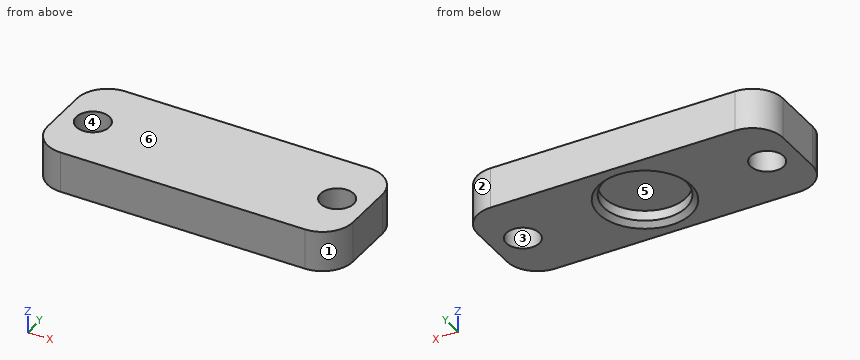
from build123d import *

# Parameters (mm, degrees)
SKETCH1_W                        = 95.25
SKETCH1_H                        = 34.925
BASE_FLANGE1_DEPTH               = 12.7
SKETCH2_R                        = 12.827
CUT_EXTRUDE1_DEPTH               = 4.7625
F_13_32_0_40625_DIAMETER_HOLE1_D = 10.31875
CHAMFER1_SIZE                    = 1.5875
FILLET1_R                        = 9.525


# Sheet-metal steps are written as plain solids
with BuildPart() as part:
    # Sketch1 → Base-Flange1 (new body)
    with BuildSketch(Plane.XY):
        Rectangle(SKETCH1_W, SKETCH1_H)
    extrude(amount=BASE_FLANGE1_DEPTH)

    # Sketch2 → Cut-Extrude1 (cut)
    with BuildSketch(Plane.XY):
        with Locations(Location((0, 0, 0), (0, 0, 180))):
            Circle(SKETCH2_R)
    extrude(amount=CUT_EXTRUDE1_DEPTH, mode=Mode.SUBTRACT)

    # 13/32 (0.40625) Diameter Hole1 (through all)
    with Locations(Plane.XY.offset(12.7)):
        with Locations((38.1, 0), (-38.1, 0)):
            Hole(F_13_32_0_40625_DIAMETER_HOLE1_D / 2)

    # Chamfer1
    chamfer1_edges = [part.edges().sort_by_distance(p)[0] for p in [
        (12.827, 0, 0),
    ]]
    chamfer(chamfer1_edges, length=CHAMFER1_SIZE)

    # Fillet1
    fillet1_edges = [part.edges().sort_by_distance(p)[0] for p in [
        (-47.625, 17.4625, 6.35),
        (47.625, 17.4625, 6.35),
        (47.625, -17.4625, 6.35),
        (-47.625, -17.4625, 6.35),
    ]]
    fillet(fillet1_edges, radius=FILLET1_R)


solid = part.part
The listing builds one solid part. Answer for the finished solid, in the listing's coordinates (mm). Face numbers are marked on the shaded views. A direction names the side the tool comes from. Coordinates: 2 decimals unless noted, no trailing zeros. Write each loop counter-clockwise with the first axis right and the second up, starting at its lowest first coordinate (ties: lowest second). Pieces come first, ordered by that corner, then holes. Notation, with made-up numbers: M 51.5,-30 L 101.5,-30 A9 ccw 101.5,-14 Z; hole C -2.75,11 d1. An arc over 180 degrees is marked long. Write each question's results on one line, items separated by ' | '.
Item 1: For a pull along Y with two mould halves and no side action, classify the marked faces 1, 2, 3 and 4 as released by +Y, released by -Y, zero draft, split by the parting line, or undercut.
Answer below:
face 1: released by -Y | face 2: released by +Y | face 3: undercut | face 4: undercut
Item 2: Consider probe 1 along Y at (x, z) = (-38.1, 8.5); probe 2 along Y at (x, z) = (0, 3.4); probe 3 along X at (y, z) = (4, 3.25) (3 decimals). Determine where each line is inside the solid, lowest interval first. Write a range as [from, to].
Answer below:
probe 1: [-17.46, -5.16], [5.16, 17.46] | probe 2: [-17.46, -12.83], [12.83, 17.46] | probe 3: [-47.625, -41.359], [-34.841, -12.187], [12.187, 34.841], [41.359, 47.625]
Item 3: Given P1, Ø7.5, axis at x = 0, y = -5, coming from the -Z side; P2, Ø8.5, axis at x = -38.1, y = 0, coming from the -Z side, each flat-ended and moving along its own axis, determine where each tip first touches the part or whether it passes through.
Answer below:
P1: z = 4.76 | P2: through
Item 4: Which of the six approach directions +Z, -Z, +X, -X, +Y, -Y give full straight-line access (tool end or side, diameter ignored) to the marked faces 5 and 6?
Answer below:
face 5: -Z | face 6: +Z, +X, -X, +Y, -Y
Item 5: The part is cut by section C-C on x = 0. Determine the outline of the cut face in (y, z), and give its area (3 significant figures).
Answer below:
outline: M -17.46,0 L -14.41,0 L -12.83,1.59 L -12.83,4.76 L 12.83,4.76 L 12.83,1.59 L 14.41,0 L 17.46,0 L 17.46,12.7 L -17.46,12.7 Z | area: 319 mm2
Item 6: The part is cut by section A-A on y = 0. Determine the outline of the cut face in (x, z) (1 decimal).
Answer below:
outline: M -47.6,0 L -43.3,0 L -43.3,12.7 L -47.6,12.7 Z; M -32.9,0 L -14.4,0 L -12.8,1.6 L -12.8,4.8 L 12.8,4.8 L 12.8,1.6 L 14.4,0 L 32.9,0 L 32.9,12.7 L -32.9,12.7 Z; M 43.3,0 L 47.6,0 L 47.6,12.7 L 43.3,12.7 Z
Item 7: The part is cut by section B-B on z = 8.5. State how many separate pieces and enclosed holes the cut face has, and give its area (3 significant figures).
Answer below:
separate pieces: 1 | enclosed holes: 2 | area: 3,080 mm2
